Can you work these out from the model? Positions are in its coordinate system, mm. A direction names the side the tool comes from. Round coordinates to 2 decimals unless told otherwise and drop trailing zeros. Order: outer loops, then holes, each group sorted by start corner. A loop starts at its lowest first (then second) coordinate and runs counter-clockwise, first axis right, second up. Notation, with made-up numbers: (68.25, 89) -> (114.25, 89) arc R21 cw to (114.25, 97) -> close; hole circle Ø9 at (31, 59). An arc over 180 degrees is marked (long way). Use a Markdown table: item, result. Add a question column.
Q1. For faces 5 (the face through (-34, -6, 10)), 6 (the face through (-48, -6, 7)), which set-ups out of +Z, -Z, +X, -X, +Y, -Y let a thin tool reach every point of the face, with its end or its side?
Q2. I'm going to push a flat-ended pin straight in: pin 1 Ø3 at (x, y) = (-47.95, -6.43) entering from -Z. Where does the tip first touch, or does it pass through?
Q3. If we section it at B-B on x = -17: List the corners of the cut face in (y, z) for me.
Q4. If we section it at A-A on z = 2.25: List the corners of the cut face in (x, y) for me, plus the area to 3 significant figures.
Q5. I need wall thicknesses on line 1 along X through (y, z) = (-6.25, 5.5); line 2 along X through (y, z) = (-7.25, 4.25); line 3 along Y through (x, z) = (-49.5, 3.25). Which ranges of each line are inside material? Lowest first, please. Write a range as [from, to].
Q6. If we section it at C-C on x = -48: List the corners of the cut face in (y, z) for me.
Q7. We'd pull the mould along Y, two halves only. Please class faces 1 (the face through (-53.445, -6, 5)), 2 (the face through (-50.01, -4.85, 3.45)), 3 (the face through (-34, -1.429, 5)), 4 (the face through (-33, -11.429, 5)): +Y half, -Y half, draft (parallel to the pull), parting line (faces both ways), or undercut.
Autodesk Inventor part; units mm, degrees
ref_plane "YZ Plane" through (0, 0, 0) normal (1, 0, 0) x (0, 1, 0)
ref_plane "XZ Plane" through (0, 0, 0) normal (0, 1, 0) x (-1, 0, 0)
ref_plane "XY Plane" through (0, 0, 0) normal (0, 0, 1) x (1, 0, 0)
sketch "Sketch1" plane through (0, 0, 0) normal (0, 0, 1) x (1, 0, 0)
  line L0 (-53.4454, -1.4286) -> (-13.4454, -1.4286)
  line L1 (-13.4454, -1.4286) -> (-13.4454, -11.4286)
  line L2 (-13.4454, -11.4286) -> (-53.4454, -11.4286)
  line L3 (-53.4454, -11.4286) -> (-53.4454, -1.4286)
  circle A0 centre (-47.9454, -6.4286) radius 2.6
  circle A1 centre (-18.9454, -6.4286) radius 2.6
  point P0 (0, 0)
  dimension "d0" = 10
  dimension "d1" = 5.2
  dimension "d2" = 5.2
  dimension "d3" = 5
  dimension "d4" = 5
  dimension "d5" = 40
  dimension "d6" = 5.5
  dimension "d7" = 34.5
extrude "Extrusion1" add sketch "Sketch1" along normal blind 7
sketch "Sketch2" plane through (0, 0, 7) normal (0, 0, 1) x (1, 0, 0)
  line L0 (-53.4454, -1.4286) -> (-13.4454, -1.4286)
  line L1 (-13.4454, -1.4286) -> (-13.4454, -11.4286)
  line L2 (-13.4454, -11.4286) -> (-53.4454, -11.4286)
  line L3 (-53.4454, -11.4286) -> (-53.4454, -1.4286)
  point P0 (0, 0)
extrude "Extrusion2" add sketch "Sketch2" along normal blind 3
properties part number "Tubebase"
Answer below:
| question | item | result |
|---|---|---|
| 1 | face 5 | +Z, +X, -X, +Y, -Y |
| 1 | face 6 | -Z |
| 2 | pin 1 | z = 7 |
| 3 | outline | (-11.43, 0) -> (-8.15, 0) -> (-8.15, 7) -> (-4.7, 7) -> (-4.7, 0) -> (-1.43, 0) -> (-1.43, 10) -> (-11.43, 10) -> close |
| 4 | outline | (-53.45, -11.43) -> (-13.45, -11.43) -> (-13.45, -1.43) -> (-53.45, -1.43) -> close; hole circle Ø5.2 at (-47.95, -6.43); hole circle Ø5.2 at (-18.95, -6.43) |
| 4 | area | 358 mm² |
| 5 | line 1 | [-53.45, -50.54], [-45.35, -21.54], [-16.35, -13.45] |
| 5 | line 2 | [-53.45, -50.41], [-45.48, -21.41], [-16.48, -13.45] |
| 5 | line 3 | [-11.43, -8.51], [-4.34, -1.43] |
| 6 | outline | (-11.43, 0) -> (-9.03, 0) -> (-9.03, 7) -> (-3.83, 7) -> (-3.83, 0) -> (-1.43, 0) -> (-1.43, 10) -> (-11.43, 10) -> close |
| 7 | face 1 | draft |
| 7 | face 2 | undercut |
| 7 | face 3 | +Y half |
| 7 | face 4 | -Y half |
